For this review, take the finished solid that the model builds, in its own axes (mm). A direction names the side the tool comes from. Give positions to 0.01 mm unless a question says otherwise; leave off trailing zeros. Order: outer loops, then holes, each group sorted by start corner. A loop starts at its lowest first (then second) coordinate and runs counter-clockwise, first axis right, second up. Notation, with made-up numbers: (-25.75, 25.25) -> (-9.75, 25.25) arc R15 cw to (-9.75, 29.25) -> close; hole circle Ø5 at (6, 14). An arc over 180 degrees is marked (long way). One line per item, written item: value. Start each with the question number.
from build123d import *

# Parameters (mm, degrees)
F0_W     = 15
F0_H     = 15.2
F0_R     = 1.725
F1_DEPTH = 4
F3_DEPTH = 66
F5_DEPTH = 2
F6_DEPTH = 4
F7_SIZE2 = 11.2
F7_SIZE  = 66
F8_R     = 2


with BuildPart() as f1:
    # F0 (on Top) → F1 (new body)
    with BuildSketch(Plane.XY):
        Rectangle(F0_W, F0_H)
        with Locations((0, -2)):
            Circle(F0_R, mode=Mode.SUBTRACT)
    extrude(amount=F1_DEPTH)

    # F2 (on face) → F3 (join)
    with BuildSketch(Plane.XY.offset(4)):
        Polygon((-7.5, 7.6), (-7.5, -7.6), (-3.5, -7.6), (-3.5, -2), (-3.5, 3.6), (3.5, 3.6), (3.5, -2), (3.5, -7.6), (7.5, -7.6), (7.5, 7.6), align=None)
    extrude(amount=F3_DEPTH)

    # F4 (on face) → F5 (cut)
    with BuildSketch(Plane.XZ.offset(-3.6)):
        with BuildLine():
            Line((-1.725, 13.045385854), (-1.725, 61.954614146))
            ThreePointArc((-1.725, 61.954614146), (-3.0238634228, 63.2375443268), (-3.5, 65))
            Line((-3.5, 65), (-3.5, 10.0000000135))
            ThreePointArc((-3.5, 10.0000000135), (-3.0238634194, 11.762455679), (-1.725, 13.045385854))
        make_face()
        with BuildLine():
            ThreePointArc((3.5, 65), (3.0238634228, 63.2375443268), (1.725, 61.954614146))
            Line((1.725, 61.954614146), (1.725, 13.045385854))
            ThreePointArc((1.725, 13.045385854), (3.0238634228, 11.7624556732), (3.5, 10))
            Line((3.5, 10), (3.5, 65))
        make_face()
        with BuildLine():
            ThreePointArc((-1.725, 65), (0, 66.725), (1.725, 65))
            Line((1.725, 65), (1.725, 61.954614146))
            ThreePointArc((1.725, 61.954614146), (3.0238634228, 63.2375443268), (3.5, 65))
            ThreePointArc((3.5, 65), (0, 68.5), (-3.5, 65))
            ThreePointArc((-3.5, 65), (-3.0238634228, 63.2375443268), (-1.725, 61.954614146))
            Line((-1.725, 61.954614146), (-1.725, 65))
        make_face()
        with BuildLine():
            ThreePointArc((3.5, 10), (3.0238634228, 11.7624556732), (1.725, 13.045385854))
            Line((1.725, 13.045385854), (1.725, 10))
            ThreePointArc((1.725, 10), (0, 8.275), (-1.725, 10))
            Line((-1.725, 10), (-1.725, 13.045385854))
            ThreePointArc((-1.725, 13.045385854), (-3.0238634194, 11.762455679), (-3.5, 10.0000000135))
            ThreePointArc((-3.5, 10.0000000135), (-6.7e-09, 6.5), (3.5, 10))
        make_face()
    extrude(amount=-F5_DEPTH, mode=Mode.SUBTRACT)

    # F4 (on face) → F6 (cut, through all)
    with BuildSketch(Plane.XZ.offset(-3.6)):
        with BuildLine():
            ThreePointArc((-1.725, 65), (0, 63.275), (1.725, 65))
            ThreePointArc((1.725, 65), (0, 66.725), (-1.725, 65))
        make_face()
        with BuildLine():
            Line((1.725, 61.954614146), (1.725, 65))
            ThreePointArc((1.725, 65), (0, 63.275), (-1.725, 65))
            Line((-1.725, 65), (-1.725, 61.954614146))
            ThreePointArc((-1.725, 61.954614146), (0, 61.5), (1.725, 61.954614146))
        make_face()
        with BuildLine():
            Line((1.725, 13.045385854), (1.725, 61.954614146))
            ThreePointArc((1.725, 61.954614146), (0, 61.5), (-1.725, 61.954614146))
            Line((-1.725, 61.954614146), (-1.725, 13.045385854))
            ThreePointArc((-1.725, 13.045385854), (0, 13.5), (1.725, 13.045385854))
        make_face()
        with BuildLine():
            Line((1.725, 10), (1.725, 13.045385854))
            ThreePointArc((1.725, 13.045385854), (0, 13.5), (-1.725, 13.045385854))
            Line((-1.725, 13.045385854), (-1.725, 10))
            ThreePointArc((-1.725, 10), (0, 11.725), (1.725, 10))
        make_face()
        with BuildLine():
            ThreePointArc((-1.725, 10), (0, 8.275), (1.725, 10))
            ThreePointArc((1.725, 10), (0, 11.725), (-1.725, 10))
        make_face()
    extrude(amount=-F6_DEPTH, mode=Mode.SUBTRACT)

    # F7
    f7_edges = [f1.edges().sort_by_distance(p)[0] for p in [
        (5.5, -7.6, 70),
        (-5.5, -7.6, 70),
    ]]
    f7_side = f1.faces().sort_by_distance((-6.784109, -7.6, 35))[0]
    chamfer(f7_edges, length=F7_SIZE, length2=F7_SIZE2, reference=f7_side)

    # F8
    f8_edges = [f1.edges().sort_by_distance(p)[0] for p in [
        (-7.5, 5.6, 70),
        (7.5, 5.6, 70),
        (-7.5, 0, 0),
        (7.5, 0, 0),
    ]]
    fillet(f8_edges, radius=F8_R)


solid = f1.part
Q1. For pin 1 Ø2 at (x, y) = (-0.5, 0) entering from +Z; pin 2 Ø4 at (x, z) = (1, 68) entering from -Y; pin 3 Ø5.5 at (x, z) = (-0.5, 43) entering from -Y, all flat-tipped, find the tip position at first contact; note any pin that passes through.
Q2. Take a section at B-B (y = -2). State the section outline as (x, z) points (3 decimals).
Q3. Take a section at C-C (z = 30). State the section outline as (x, y) points (3 decimals), and give its area (3 significant figures).
Q4. For faces 1 (the flat face through (0, 0, 0)), 2 (the flat face through (0, 3.6, 6)), 3 (the cylindrical face through (-0.1, 4.6, 6.5)), 4 (the flat face through (-1.725, 7, 38)), 5 (the flat face through (7.5, 2, 27)), list the 3-axis set-ups (+Z, -Z, +X, -X, +Y, -Y) from which the entire face can be reached by the end or side of a thin tool; tool diameter is ignored.
Q5. For line 1 along X through (y, z) = (1, 36); line 2 along Y through (x, z) = (0, 3) (3 decimals); line 3 along X through (y, z) = (6.75, 25.5) (3 decimals), list the stretches that pass through material, from the lowest coordinate up.
Q6. Mouldability with a two-part tool opening along X and no side actions: class faces 6 (the flat face through (-2, 5.6, 38)), 7 (the flat face through (5, -2, 37)), 8 (the cylindrical face through (-6.93, 0.11, 0.6)) as pulls with the +X half, pulls with the -X half, needs draft (parallel to the pull), parting line crosses it, or undercut.
Q7. Take a section at A-A (x = 0). State the section outline as (y, z) points (3 decimals), and give its area (3 significant figures).
Q8. Take a section at D-D (y = 1). State the section outline as (x, z) points.
Answers below:
1. pin 1: stops at z = 4
1. pin 2: stops at y = 3.6
1. pin 3: stops at y = 5.6
2. outline: (-7.5, 2) arc R2 ccw to (-5.5, 0) -> (-1.725, 0) -> (-1.725, 4) -> (-3.5, 4) -> (-3.5, 37) -> (-7.5, 37) -> close; (1.725, 0) -> (5.5, 0) arc R2 ccw to (7.5, 2) -> (7.5, 37) -> (3.5, 37) -> (3.5, 4) -> (1.725, 4) -> close
3. outline: (-7.5, -3.188) -> (-3.5, -3.188) -> (-3.5, 5.6) -> (-1.725, 5.6) -> (-1.725, 7.6) -> (-7.5, 7.6) -> close; (1.725, 5.6) -> (3.5, 5.6) -> (3.5, -3.188) -> (7.5, -3.188) -> (7.5, 7.6) -> (1.725, 7.6) -> close
3. area: 93.4 mm²
4. face 1: -Z, +X, -X, +Y, -Y
4. face 2: +Z, -Y
4. face 3: -Y
4. face 4: +Y, -Y
4. face 5: +Z, -Z, +X, +Y, -Y
5. line 1: x = -7.5 to -3.5, 3.5 to 7.5
5. line 2: y = -7.6 to -3.725, -0.275 to 7.6
5. line 3: x = -7.5 to -1.725, 1.725 to 7.5
6. face 6: undercut
6. face 7: needs draft
6. face 8: pulls with the -X half
7. outline: (-7.6, 0) -> (-3.725, 0) -> (-3.725, 4) -> (-7.6, 4) -> close; (-0.275, 0) -> (7.6, 0) -> (7.6, 8.275) -> (5.6, 8.275) -> (5.6, 6.5) -> (3.6, 6.5) -> (3.6, 4) -> (-0.275, 4) -> close; (3.6, 68.5) -> (5.6, 68.5) -> (5.6, 66.725) -> (7.6, 66.725) -> (7.6, 70) -> (3.6, 70) -> close
7. area: 70.1 mm²
8. outline: (-7.5, 2) arc R2 ccw to (-5.5, 0) -> (5.5, 0) arc R2 ccw to (7.5, 2) -> (7.5, 54.68) -> (3.5, 54.68) -> (3.5, 4) -> (-3.5, 4) -> (-3.5, 54.68) -> (-7.5, 54.68) -> close
